Work out the finished part from the listing and answer in its coordinate system (mm). Face numbers are marked on the shaded views. A direction names the side the tool comes from. Give positions to 0.01 mm unless a question says otherwise; leave off trailing zeros. Order: outer loops, then holes, each group sorted by start corner. A loop starts at its lowest first (then second) coordinate and runs counter-clockwise, first axis right, second up. Notation, with made-up numbers: (42, 52) - (79, 52) arc R14 cw to (79, 69) - close; hole circle Ø8 at (46.5, 79). An arc over 180 degrees is marked (long way). Put each result on its own line as item: value.
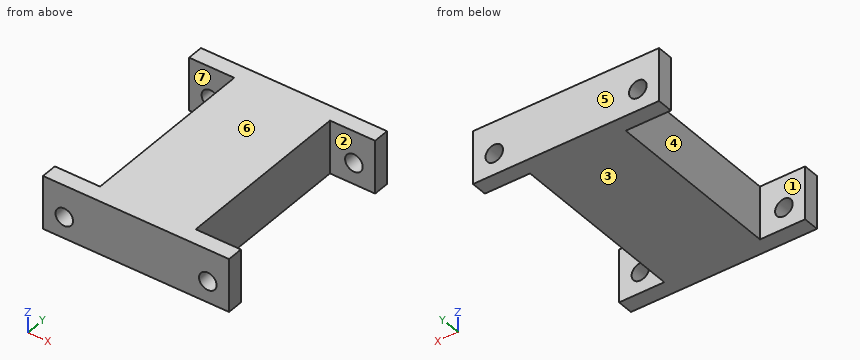
```python
from build123d import *

# Parameters (mm, degrees)
SKETCH1_W           = 35
SKETCH1_H           = 10
BOSS_EXTRUDE1_DEPTH = 1.5
SKETCH2_R           = 1.65
CUT_EXTRUDE1_DEPTH  = 3
SKETCH3_W           = 18
SKETCH3_H           = 10
BOSS_EXTRUDE2_DEPTH = 34


with BuildPart() as part:
    # Sketch1 → Boss-Extrude1 (new body, symmetric)
    with BuildSketch(Plane(origin=(0, 0, 0), x_dir=(1, 0, 0), z_dir=(0, 1, 0))):
        Rectangle(SKETCH1_W, SKETCH1_H)
    boss_extrude1 = extrude(amount=BOSS_EXTRUDE1_DEPTH, both=True)

    # Sketch2 → Cut-Extrude1 (cut)
    with BuildSketch(Plane(origin=(0, 1.5, 0), x_dir=(1, 0, 0), z_dir=(0, 1, 0))):
        with Locations((-13.5, 1)):
            Circle(SKETCH2_R)
        with Locations((13.5, 1)):
            Circle(SKETCH2_R)
    cut_extrude1 = extrude(amount=-CUT_EXTRUDE1_DEPTH, mode=Mode.SUBTRACT)

    # Sketch3 → Boss-Extrude2 (add)
    with BuildSketch(Plane(origin=(0, 1.5, 0), x_dir=(1, 0, 0), z_dir=(0, 1, 0))):
        Rectangle(SKETCH3_W, SKETCH3_H)
    extrude(amount=BOSS_EXTRUDE2_DEPTH)

    # Mirror1: Boss-Extrude1, Cut-Extrude1 across plane
    add(boss_extrude1.mirror(Plane.ZX.offset(18.5)))
    add(cut_extrude1.mirror(Plane.ZX.offset(18.5)), mode=Mode.SUBTRACT)


solid = part.part
```
(1) Determine the mould class of the marked faces 4, 5, 6 and 7 for opening direction Y: pulls with the +Y half, pulls with the -Y half, needs draft (parallel to the pull), parting line crosses it, or undercut.
Geometry check:
face 4: undercut
face 5: pulls with the +Y half
face 6: needs draft
face 7: undercut
(2) Section C-C, the plane z = -3.25 is taken. Write down the section's boundary in (x, y).
Geometry check:
outline: (-17.5, -1.5) - (17.5, -1.5) - (17.5, 1.5) - (9, 1.5) - (9, 35.5) - (17.5, 35.5) - (17.5, 38.5) - (-17.5, 38.5) - (-17.5, 35.5) - (-9, 35.5) - (-9, 1.5) - (-17.5, 1.5) - close
(3) Given pin 1 (2.5 mm diameter, centred on x = 13.5, z = -1, fed in from -Y); pin 2 (3 mm diameter, centred on y = 17, z = -1.5, fed in from -X); pin 3 (3 mm diameter, centred on y = 25.5, z = 2, fed in from +X), each flat-ended and moving along its own axis, determine where each tip first touches the part or whether it passes through.
Geometry check:
pin 1: passes through
pin 2: stops at x = -9
pin 3: stops at x = 9
(4) Section A-A, the plane x = 13.5 is taken. Write down the section's boundary in (y, z).
Geometry check:
outline: (-1.5, -5) - (1.5, -5) - (1.5, -2.65) - (-1.5, -2.65) - close; (-1.5, 0.65) - (1.5, 0.65) - (1.5, 5) - (-1.5, 5) - close; (35.5, -5) - (38.5, -5) - (38.5, -2.65) - (35.5, -2.65) - close; (35.5, 0.65) - (38.5, 0.65) - (38.5, 5) - (35.5, 5) - close
(5) Straight lines are drawn through the part: line 1 (X direction, y = 36.35, z = -1); line 2 (Y direction, x = -15, z = -2); line 3 (Z direction, x = 13.5, y = 36.4). For each, find the intervals that lie inside material, in ascending order.
Geometry check:
line 1: x = -17.5 to -15.15, -11.85 to 11.85, 15.15 to 17.5
line 2: y = -1.5 to 1.5, 35.5 to 38.5
line 3: z = -5 to -2.65, 0.65 to 5
(6) Section D-D, the plane y = 10.5 is taken. Write down the section's boundary in (x, z).
Geometry check:
outline: (-9, -5) - (9, -5) - (9, 5) - (-9, 5) - close
(7) Section B-B, the plane z = -1 is taken. Write down the section's boundary in (x, y), then the cut area to 3 significant figures.
Geometry check:
outline: (-17.5, -1.5) - (-15.15, -1.5) - (-15.15, 1.5) - (-17.5, 1.5) - close; (-17.5, 35.5) - (-15.15, 35.5) - (-15.15, 38.5) - (-17.5, 38.5) - close; (-11.85, -1.5) - (11.85, -1.5) - (11.85, 1.5) - (9, 1.5) - (9, 35.5) - (11.85, 35.5) - (11.85, 38.5) - (-11.85, 38.5) - (-11.85, 35.5) - (-9, 35.5) - (-9, 1.5) - (-11.85, 1.5) - close; (15.15, -1.5) - (17.5, -1.5) - (17.5, 1.5) - (15.15, 1.5) - close; (15.15, 35.5) - (17.5, 35.5) - (17.5, 38.5) - (15.15, 38.5) - close
area: 782 mm²
(8) A tool of negligible diameter and unlimited length cuts with its end or side. For the marked faces 1, 2 and 3, from which of +Z, -Z, +X, -X, +Y, -Y can it reach the whole face along a straight path? Write none if from no direction.
Geometry check:
face 1: +Z, -Z, -X
face 2: +Z, -Z, +X
face 3: -Z, +X, -X, +Y, -Y
